Geometry check sheet. Reference: drawing and pictorial views, mm from the part's lowest x, y, z. Coordinates: 2 decimals unless noted, no trailing zeros. Loops run counter-clockwise (first coordinate to the right, second up) from the corner with the lowest first, then second, coordinate; pieces in that order, holes last. Notation, with made-up numbers: (-19.5, 67) - (22.5, 67) arc R27 cw to (22.5, 94) - close; hole circle Ø11 at (4.5, -36). An arc over 180 degrees is marked (long way). Use a Markdown table: item, result. Add a question column.
1) Sectioned sample at B-B, the plane y = 16.5. Enter the section's corners in (x, z).
2) Sectioned sample at C-C, the plane z = 4.1. Enter the section's corners in (x, y) (3 decimals), then the cut area to 3 significant figures.
3) Draft check along Y on the marked faces 1, 2 and 3. Enter one of: pulls with the +Y half, pulls with the -Y half, needs draft (parallel to the pull), parting line crosses it, or undercut.
4) Sectioned sample at D-D, the plane x = 51. Enter the section's corners in (y, z), then the cut area to 3 significant figures.
5) Go/stop test with a flat-tipped pin: P1, Ø12, axis at x = 60, y = 9.5, coming from the +Z side. Record where the tip stops, or that it passes through.
6) Sectioned sample at A-A, the plane x = 41. Enter the section's corners in (y, z), then the cut area to 3 significant figures.
7) Thickness scan on line 1 (Y direction, x = 13, z = 3.5); line 2 (X direction, y = 17, z = 1.55); line 3 (Z direction, x = 13, y = 20.5). Record the ranges inside material, lowest first.
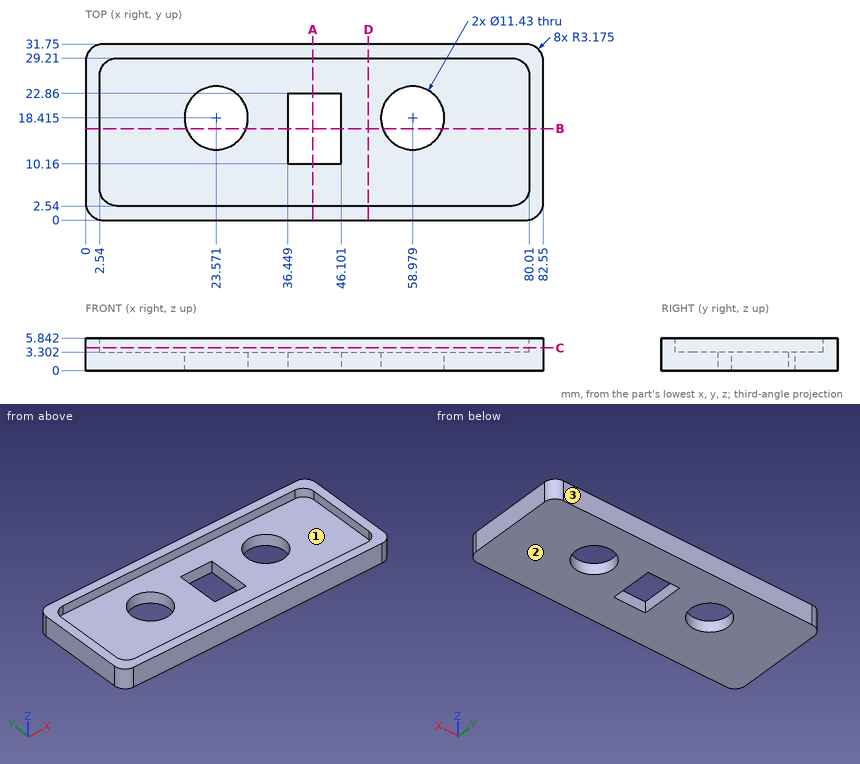
Solved:
| question | item | result |
|---|---|---|
| 1 | outline | (0, 0) - (18.19, 0) - (18.19, 3.3) - (2.54, 3.3) - (2.54, 5.84) - (0, 5.84) - close; (28.96, 0) - (36.45, 0) - (36.45, 3.3) - (28.96, 3.3) - close; (46.1, 0) - (53.59, 0) - (53.59, 3.3) - (46.1, 3.3) - close; (64.36, 0) - (82.55, 0) - (82.55, 5.84) - (80.01, 5.84) - (80.01, 3.3) - (64.36, 3.3) - close |
| 2 | outline | (0, 3.175) arc R3.175 ccw to (3.175, 0) - (79.375, 0) arc R3.175 ccw to (82.55, 3.175) - (82.55, 28.575) arc R3.175 ccw to (79.375, 31.75) - (3.175, 31.75) arc R3.175 ccw to (0, 28.575) - close; hole (2.54, 5.715) arc R3.175 ccw to (5.715, 2.54) - (76.835, 2.54) arc R3.175 ccw to (80.01, 5.715) - (80.01, 26.035) arc R3.175 ccw to (76.835, 29.21) - (5.715, 29.21) arc R3.175 ccw to (2.54, 26.035) - close |
| 2 | area | 555 mm2 |
| 3 | face 1 | undercut |
| 3 | face 2 | needs draft |
| 3 | face 3 | pulls with the +Y half |
| 4 | outline | (0, 0) - (31.75, 0) - (31.75, 5.84) - (29.21, 5.84) - (29.21, 3.3) - (2.54, 3.3) - (2.54, 5.84) - (0, 5.84) - close |
| 4 | area | 118 mm2 |
| 5 | P1 | stops at z = 3.3 |
| 6 | outline | (0, 0) - (10.16, 0) - (10.16, 3.3) - (2.54, 3.3) - (2.54, 5.84) - (0, 5.84) - close; (22.86, 0) - (31.75, 0) - (31.75, 5.84) - (29.21, 5.84) - (29.21, 3.3) - (22.86, 3.3) - close |
| 6 | area | 75.8 mm2 |
| 7 | line 1 | y = 0 to 2.54, 29.21 to 31.75 |
| 7 | line 2 | x = 0 to 18.03, 29.11 to 36.45, 46.1 to 53.44, 64.52 to 82.55 |
| 7 | line 3 | z = 0 to 3.3 |
